from build123d import *

# Parameters (mm, degrees)
SKETCH_W      = 35
SKETCH_H      = 40
EXTRUDE_DEPTH = 3


with BuildPart() as part:
    # Sketch → Extrude (new body)
    with BuildSketch(Plane.XY):
        Rectangle(SKETCH_W, SKETCH_H)
        Polygon((-7.5, -7.5), (-7.5, 7.5), (7.5, 7.5), (7.5, 3.5), (12.5, 3.5), (12.5, -3.5), (7.5, -3.5), (7.5, -7.5), align=None, mode=Mode.SUBTRACT)
    extrude(amount=EXTRUDE_DEPTH)


solid = part.part
Check sheet for the modelled part. Datum: model origin and axes. Units: mm. A direction names the side the tool comes from. Give positions to 0.01 mm unless a question says otherwise; leave off trailing zeros. Loops run counter-clockwise (first coordinate to the right, second up) from the corner with the lowest first, then second, coordinate; pieces in that order, holes last. Notation, with made-up numbers: M -29,-9.5 L -19,-9.5 A8 ccw -19,-3.5 Z; hole C -37,-17 d7. An arc over 180 degrees is marked long. Return JSON: item names as keys, results as strings. Group by question number.
1. Cross-section at A-A on y = -5.5. Record the boundary of the cut face in (x, z).
2. Tool access check on faces 4 (the flat face through (0, 20, 1)), 5 (the flat face through (-7.5, 0, 1)). Record the directions out of +Z, -Z, +X, -X, +Y, -Y that give a thin tool (end or side, any length) a straight path to the whole face; none if there is none.
3. Cross-section at C-C on z = 0.95. Record the boundary of the cut face in (x, y), plus the area to 3 significant figures.
4. Cross-section at B-B on x = 9. Record the boundary of the cut face in (y, z).
5. Mould release check, pull along X, two halves, no side actions. Record for faces 1 (the flat face through (-8, 0, 3)), 2 (the flat face through (17.5, 0, 1)), 3 (the flat face through (0, 7.5, 1)): released by +X, released by -X, zero draft, split by the parting line, or undercut.
6. Thickness scan on L1, parallel to X at y = -4.5, z = 1.8; L2, parallel to X at y = -3, z = 1.9; L3, parallel to Y at x = 11, z = 1.7. Record the ranges inside material, lowest first.
Return value:
{
 "1": {"outline": "M -17.5,0 L -7.5,0 L -7.5,3 L -17.5,3 Z; M 7.5,0 L 17.5,0 L 17.5,3 L 7.5,3 Z"},
 "2": {"face 4": "+Z, -Z, +X, -X, +Y", "face 5": "+Z, -Z"},
 "3": {"outline": "M -17.5,-20 L 17.5,-20 L 17.5,20 L -17.5,20 Z; hole M -7.5,-7.5 L 7.5,-7.5 L 7.5,-3.5 L 12.5,-3.5 L 12.5,3.5 L 7.5,3.5 L 7.5,7.5 L -7.5,7.5 Z", "area": "1,140 mm^2"},
 "4": {"outline": "M -20,0 L -3.5,0 L -3.5,3 L -20,3 Z; M 3.5,0 L 20,0 L 20,3 L 3.5,3 Z"},
 "5": {"face 1": "zero draft", "face 2": "released by +X", "face 3": "undercut"},
 "6": {"L1": "-17.5 to -7.5, 7.5 to 17.5", "L2": "-17.5 to -7.5, 12.5 to 17.5", "L3": "-20 to -3.5, 3.5 to 20"}
}
